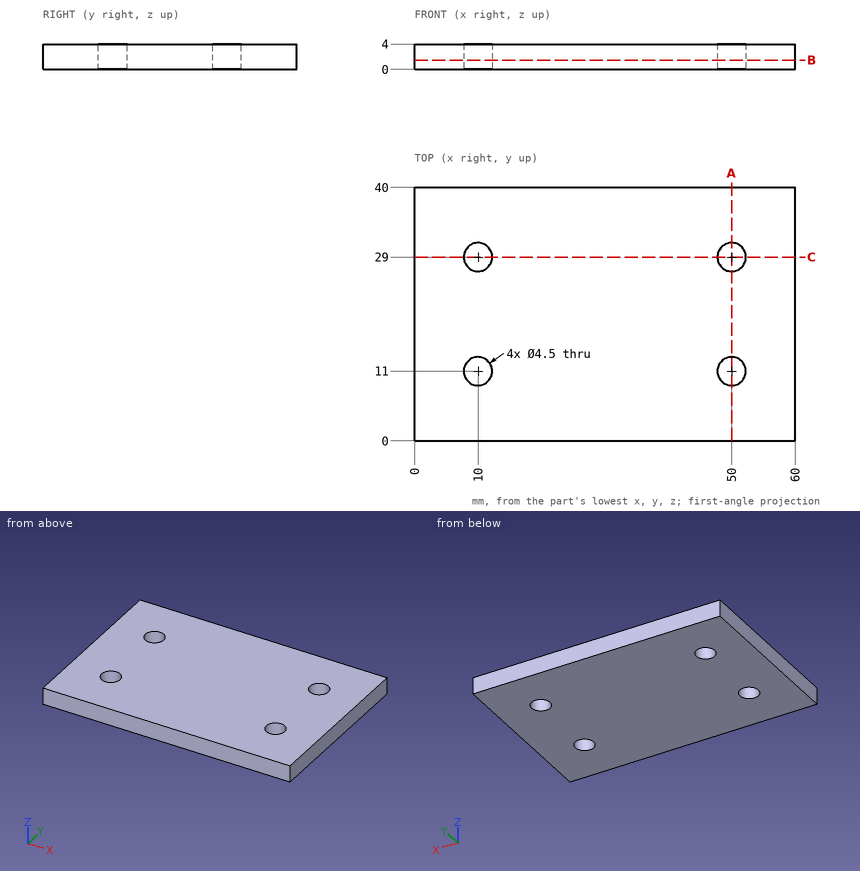
Could you check a few things on this drawing? It's one solid part, dimensions in mm from its lowest x, y, z. Give positions to 0.01 mm unless a question says otherwise; leave off trailing zeros. Order: outer loops, then holes, each group sorted by start corner. A loop starts at its lowest first (then second) coordinate and runs counter-clockwise, first axis right, second up.
1. Suppose I cut it at A-A (x = 50). Write out the boundary of the cut face in (y, z), plus the area to 3 significant figures.
Answers below:
outline: (0, 0) - (8.75, 0) - (8.75, 4) - (0, 4) - close; (13.25, 0) - (26.75, 0) - (26.75, 4) - (13.25, 4) - close; (31.25, 0) - (40, 0) - (40, 4) - (31.25, 4) - close
area: 124 mm2
2. I need wall thicknesses on L1, parallel to Y at x = 50, z = 2.7; L2, parallel to X at y = 9.5, z = 0.8; L3, parallel to Y at x = 49, z = 1.8. Which ranges of each line are inside material? Lowest first, please.
Answers below:
L1: y = 0 to 8.75, 13.25 to 26.75, 31.25 to 40
L2: x = 0 to 8.32, 11.68 to 48.32, 51.68 to 60
L3: y = 0 to 8.98, 13.02 to 26.98, 31.02 to 40
3. Suppose I cut it at C-C (y = 29). Write out the boundary of the cut face in (x, z), plus the area to 3 significant figures.
Answers below:
outline: (0, 0) - (7.75, 0) - (7.75, 4) - (0, 4) - close; (12.25, 0) - (47.75, 0) - (47.75, 4) - (12.25, 4) - close; (52.25, 0) - (60, 0) - (60, 4) - (52.25, 4) - close
area: 204 mm2
4. For pin 1 (3.5 mm diameter, centred on x = 50, y = 11, fed in from -Z), with a flat end and sliding along its axis, tell me the tip position at first contact or that it passes through.
Answers below:
pin 1: passes through
5. Suppose I cut it at B-B (z = 1.45). Write out the boundary of the cut face in (x, y).
Answers below:
outline: (0, 0) - (60, 0) - (60, 40) - (0, 40) - close; hole circle Ø4.5 at (10, 11); hole circle Ø4.5 at (10, 29); hole circle Ø4.5 at (50, 11); hole circle Ø4.5 at (50, 29)
